Autodesk Inventor part; units mm, degrees
ref_plane "YZ Plane" through (0, 0, 0) normal (1, 0, 0) x (0, 1, 0)
ref_plane "XZ Plane" through (0, 0, 0) normal (0, 1, 0) x (-1, 0, 0)
ref_plane "XY Plane" through (0, 0, 0) normal (0, 0, 1) x (1, 0, 0)
sketch "Sketch1" plane through (0, 0, 0) normal (0, 1, 0) x (-1, 0, 0)
  arc A0 (9, -27.5) -> (21, -27.5) centre (15, -27.5) ccw
  arc A1 (-9, 27.5) -> (-21, 27.5) centre (-15, 27.5) ccw
  arc A2 (21, 27.5) -> (9, 27.5) centre (15, 27.5) ccw
  arc A3 (-21, -27.5) -> (-9, -27.5) centre (-15, -27.5) ccw
  line L0 (-9, 21) -> (-9, 27.5)
  line L1 (-9, -21) -> (9, -21)
  circle A4 centre (0, 0) radius 12
  line L2 (21, -27.5) -> (21, 27.5)
  line L3 (-21, 27.5) -> (-21, -27.5)
  line L4 (9, 21) -> (-9, 21)
  line L5 (9, -21) -> (9, -27.5)
  line L6 (-9, -27.5) -> (-9, -21)
  line L7 (9, 27.5) -> (9, 21)
extrude "Extrusion1" add sketch "Sketch1" against normal blind 4.064
hole "Hole8" at (-15.5, -4.064, -15.5) direction (0, 1, 0) diameter 4 depth 4.064
hole "Hole7" at (-15.5, -4.064, 15.5) direction (0, 1, 0) diameter 4 depth 4.064
hole "Hole6" at (15.5, -4.064, 15.5) direction (0, 1, 0) diameter 4 depth 4.064
hole "Hole5" at (15.5, -4.064, -15.5) direction (0, 1, 0) diameter 4 depth 4.064
sketch "Sketch5" plane through (0, -4.064, 0) normal (0, -1, 0) x (1, 0, 0)
  point P0 (15.5, -15.5)
hole "Hole4" at (15, -4.064, -27.5) direction (0, 1, 0) diameter 4.5 depth 4.064
sketch "Sketch4" plane through (0, -4.064, 0) normal (0, -1, 0) x (1, 0, 0)
  point P0 (15.5, 15.5)
hole "Hole3" at (15, -4.064, 27.5) direction (0, 1, 0) diameter 4.5 depth 4.064
sketch "Sketch3" plane through (0, -4.064, 0) normal (0, -1, 0) x (1, 0, 0)
  point P0 (-15.5, 15.5)
hole "Hole2" at (-15, -4.064, 27.5) direction (0, 1, 0) diameter 4.5 depth 4.064
sketch "Sketch2" plane through (0, -4.064, 0) normal (0, -1, 0) x (1, 0, 0)
  point P0 (-15.5, -15.5)
hole "Hole1" at (-15, -4.064, -27.5) direction (0, 1, 0) diameter 4.5 depth 4.064
sketch "Sketch6" plane through (0, -4.064, 0) normal (0, -1, 0) x (1, 0, 0)
  point P0 (15, -27.5)
sketch "Sketch7" plane through (0, -4.064, 0) normal (0, -1, 0) x (1, 0, 0)
  point P0 (15, 27.5)
sketch "Sketch8" plane through (0, -4.064, 0) normal (0, -1, 0) x (1, 0, 0)
  point P0 (-15, 27.5)
sketch "Sketch9" plane through (0, -4.064, 0) normal (0, -1, 0) x (1, 0, 0)
  point P0 (-15, -27.5)
properties part number "Piston Motor holder" material "Aluminum 6061"
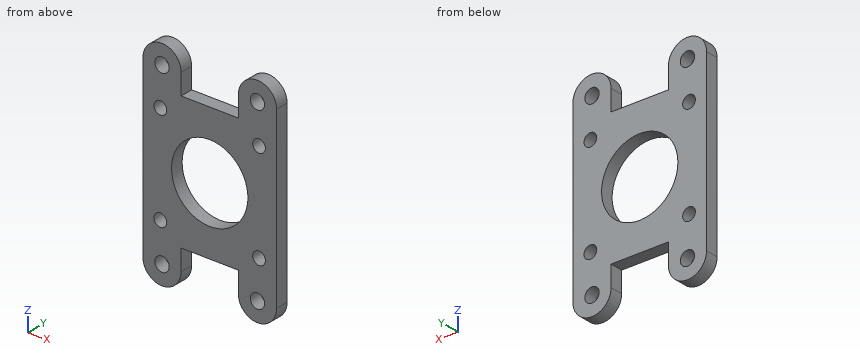
Source: CAD feature listing. Evaluate the final solid. Frame: model axes, mm. Round coordinates to 2 decimals unless told otherwise and drop trailing zeros. Loops run counter-clockwise (first coordinate to the right, second up) from the corner with the lowest first, then second, coordinate; pieces in that order, holes last. Notation, with made-up numbers: (14.25, 45) -> (51.25, 45) arc R18 cw to (51.25, 75) -> close; hole circle Ø3 at (-12.75, 11.25). An arc over 180 degrees is marked (long way). Answer as a JSON object with one key per item and string values. Group by question number.
Q1. Section query C-C (y = -3.1). State how many separate pieces and enclosed holes the cut face has, plus the area to 3 significant figures.
Q2. Section query A-A (z = 0). Output: boundary loops of the cut face in (x, y), plus the area to 3 significant figures.
Q3. Section query B-B (z = 15.5). Output: boundary loops of the cut face in (x, y), plus the area to 3 significant figures.
Q4. Section query D-D (x = 3.5). Output: boundary loops of the cut face in (y, z), plus the area to 3 significant figures.
Q5. Ray query, line 1 (X direction, y = -2.25, z = -27.5); line 2 (X direction, y = -2.95, z = 15.5); line 3 (Z direction, x = 0, y = -1.3). Return the intervals inside material, ascending. Write a range as from..to.
Q6. Contact query for flat-ended pins moving along their axis: P1, Ø6, axis at x = -7, z = -22, coming from the -Y side; P2, Ø4, axis at x = -6.5, z = 7.5, coming from the +Y side; P3, Ø1, axis at x = 5, y = -2, coming from the -Z side; P4, Ø1.2, axis at x = 1.5, y = -2, coming from the +Z side. Output: stop coordinate, or through.
Completed:
{
 "1": {"separate pieces": "1", "enclosed holes": "9", "area": "1,740 mm²"},
 "2": {"outline": "(-21, -4.06) -> (-12, -4.06) -> (-12, 0) -> (-21, 0) -> close; (12, -4.06) -> (21, -4.06) -> (21, 0) -> (12, 0) -> close", "area": "73.2 mm²"},
 "3": {"outline": "(-21, -4.06) -> (-17.5, -4.06) -> (-17.5, 0) -> (-21, 0) -> close; (-13.5, -4.06) -> (13.5, -4.06) -> (13.5, 0) -> (-13.5, 0) -> close; (17.5, -4.06) -> (21, -4.06) -> (21, 0) -> (17.5, 0) -> close", "area": "138 mm²"},
 "4": {"outline": "(-4.06, -21) -> (0, -21) -> (0, -11.48) -> (-4.06, -11.48) -> close; (-4.06, 11.48) -> (0, 11.48) -> (0, 21) -> (-4.06, 21) -> close", "area": "77.4 mm²"},
 "5": {"line 1": "-21..-17.25, -12.75..-9, 9..12.75, 17.25..21", "line 2": "-21..-17.5, -13.5..13.5, 17.5..21", "line 3": "-21..-12, 12..21"},
 "6": {"P1": "y = -4.06", "P2": "through", "P3": "z = -21", "P4": "z = 21"}
}
